Here's the drawing with two shaded views (mm, measured from the low corner). I have some questions. Round coordinates to 2 decimals unless told otherwise and drop trailing zeros. Loops run counter-clockwise (first coordinate to the right, second up) from the corner with the lowest first, then second, coordinate; pieces in that order, holes last. Notation, with made-up numbers: (9.5, -8) -> (14.5, -8) arc R12 cw to (14.5, 7) -> close; hole circle Ø11 at (-4, 65.5). An arc over 180 degrees is marked (long way). Write each question's results on one line, items separated by ' | '. Start each with the question number.
1) Imagine slicing it at C-C, the plane y = 13.5. List the corners of the cut face in (x, z) for me, plus the area to 3 significant figures.
2) Imagine slicing it at B-B, the plane z = 3.5. Give the number of separate pieces and of enclosed holes in the cut face, plus the area to 3 significant figures.
3) For P1, Ø14.5, axis at x = 80, y = 23.5, coming from the +Z side; P2, Ø4, axis at x = 30, z = 7.5, coming from the -Y side (1 decimal); P3, Ø6.5, axis at x = 77.94, y = 112.5, coming from the +Z side; P4, Ø5, axis at x = 133, z = 7, coming from the +Y side (1 decimal), each with a flat end and sliding along its axis, tell me the tip position at first contact or that it passes through.
4) Imagine slicing it at A-A, the plane y = 40.5. List the corners of the cut face in (x, z) for me.
5) If I drill on probe 1 along Y at (x, z) = (51, 5.75) (1 decimal); probe 2 along Y at (x, z) = (49, 4.5); probe 3 along X at (y, z) = (21.5, 9) (1 decimal), over which ranges is the centre line in solid material (lowest first)?
6) We'd pull the mould along X, two halves only. Please class the marked faces 1, 2, 3 and 4: pulls with the +X half, pulls with the -X half, needs draft (parallel to the pull), parting line crosses it, or undercut.
7) Imagine slicing it at D-D, the plane y = 102. List the corners of the cut face in (x, z) for me, plus the area to 3 significant figures.
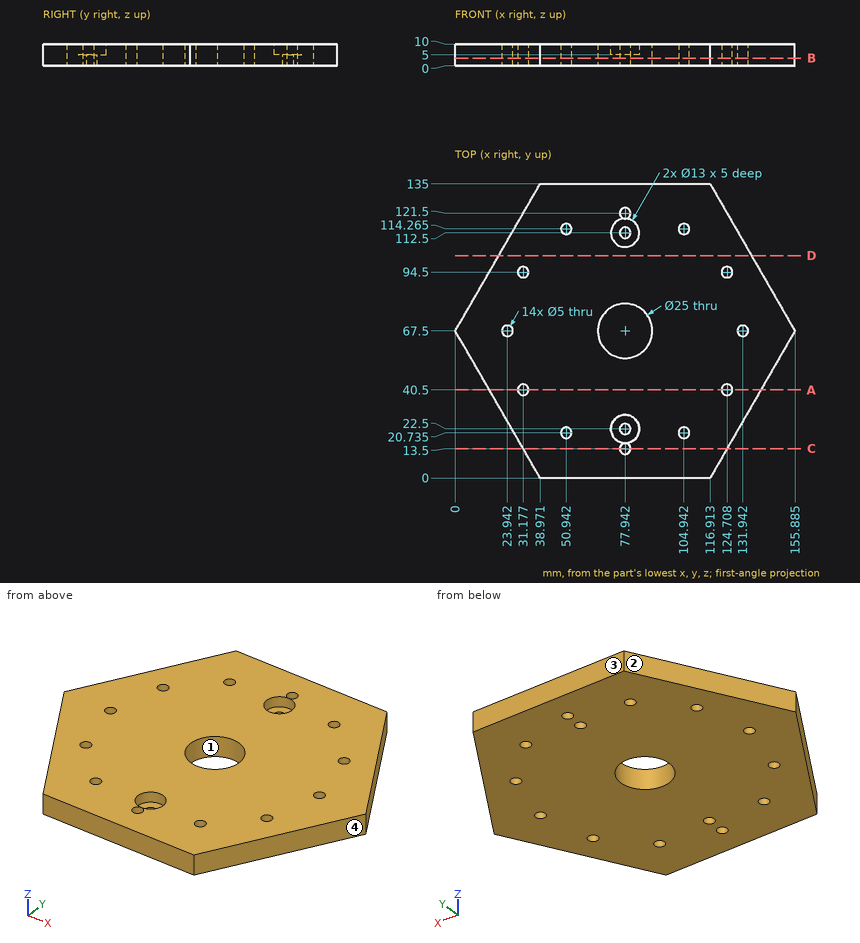
Checked values:
1) outline: (31.18, 0) -> (75.44, 0) -> (75.44, 10) -> (31.18, 10) -> close; (80.44, 0) -> (124.71, 0) -> (124.71, 10) -> (80.44, 10) -> close | area: 885 mm^2
2) separate pieces: 1 | enclosed holes: 15 | area: 15,000 mm^2
3) P1: z = 10 | P2: y = 12.1 | P3: z = 5 | P4: y = 111.5
4) outline: (15.59, 0) -> (28.68, 0) -> (28.68, 10) -> (15.59, 10) -> close; (33.68, 0) -> (122.21, 0) -> (122.21, 10) -> (33.68, 10) -> close; (127.21, 0) -> (140.3, 0) -> (140.3, 10) -> (127.21, 10) -> close
5) probe 1: 0 to 18.2, 23.2 to 111.8, 116.8 to 135 | probe 2: 0 to 19.16, 22.31 to 112.69, 115.84 to 135 | probe 3: 26.6 to 48.6, 53.3 to 71.5, 84.4 to 102.6, 107.3 to 129.3
6) face 1: undercut | face 2: pulls with the -X half | face 3: needs draft | face 4: pulls with the +X half
7) outline: (19.92, 0) -> (135.97, 0) -> (135.97, 10) -> (19.92, 10) -> close | area: 1,160 mm^2
